Could you check a few things on this model? Use its own coordinates, in mm. Face numbers are marked on the shaded views. A direction names the side the tool comes from. Coordinates: 2 decimals unless noted, no trailing zeros.
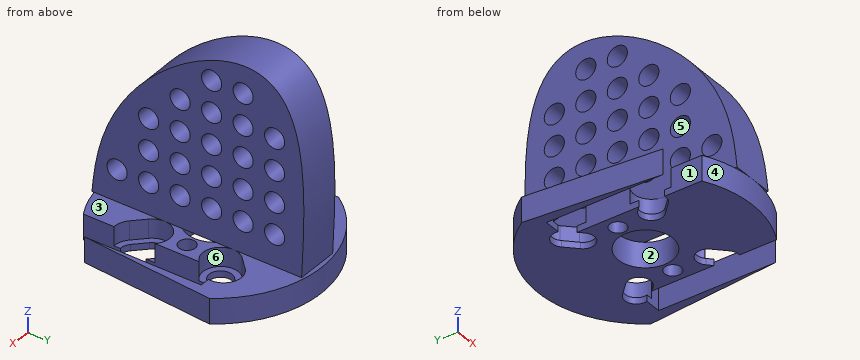
```python
from build123d import *

# Parameters (mm, degrees)
SKETCH_2_R          = 1.3
SKETCH_2_R_2        = 4.3
EXTRUDE_1_DEPTH     = 4
CUT_EXTRUDE_1_DEPTH = 3
EXTRUDE_START       = -3.4
EXTRUDE_2_DEPTH     = 6.8
CUT_EXTRUDE_START   = 3.4
SKETCH_12_R         = 1.6
CUT_EXTRUDE_2_DEPTH = 44.412015776


# Read off the part's stored shape, not the designer's step: 凸台-拉伸2
with BuildPart() as part:
    # 草图2 → 凸台-拉伸1 (new body)
    with BuildSketch(Plane.XY):
        with BuildLine():
            Line((-14.150895062, 9.420836955), (-12.3, -11.734990413))
            Line((-12.3, -11.734990413), (-12.3, 6.8))
            Line((-12.3, 6.8), (-9.717210306, 6.8))
            ThreePointArc((-9.717210306, 6.8), (-8.843521096, 8.787489117), (-6.693130483, 8.488714895))
            Line((-6.693130483, 8.488714895), (-4.92536353, 6.720947942))
            ThreePointArc((-4.92536353, 6.720947942), (-4.92536353, 4.17536353), (-7.470947942, 4.17536353))
            Line((-7.470947942, 4.17536353), (-8.2, 4.904415588))
            Line((-8.2, 4.904415588), (-8.2, -4.904415588))
            Line((-8.2, -4.904415588), (-7.470947942, -4.17536353))
            ThreePointArc((-7.470947942, -4.17536353), (-4.92536353, -4.17536353), (-4.92536353, -6.720947942))
            Line((-4.92536353, -6.720947942), (-6.693130483, -8.488714895))
            ThreePointArc((-6.693130483, -8.488714895), (-7.386916292, -8.92025587), (-8.2, -9.00063774))
            Line((-8.2, -9.00063774), (-8.2, -14.891608375))
            ThreePointArc((-8.2, -14.891608375), (0, -17), (8.2, -14.891608375))
            Line((8.2, -14.891608375), (8.2, -9.00063774))
            ThreePointArc((8.2, -9.00063774), (7.386916292, -8.92025587), (6.693130483, -8.488714895))
            Line((6.693130483, -8.488714895), (4.92536353, -6.720947942))
            ThreePointArc((4.92536353, -6.720947942), (4.92536353, -4.17536353), (7.470947942, -4.17536353))
            Line((7.470947942, -4.17536353), (8.2, -4.904415588))
            Line((8.2, -4.904415588), (8.2, 4.904415588))
            Line((8.2, 4.904415588), (7.470947942, 4.17536353))
            ThreePointArc((7.470947942, 4.17536353), (4.92536353, 4.17536353), (4.92536353, 6.720947942))
            Line((4.92536353, 6.720947942), (6.693130483, 8.488714895))
            ThreePointArc((6.693130483, 8.488714895), (8.843521096, 8.787489117), (9.717210306, 6.8))
            Line((9.717210306, 6.8), (12.3, 6.8))
            Line((12.3, 6.8), (12.3, -11.734990413))
            Line((12.3, -11.734990413), (14.150895062, 9.420836955))
            ThreePointArc((14.150895062, 9.420836955), (0, 17), (-14.150895062, 9.420836955))
        make_face()
        with Locations((-6, 0)):
            Circle(SKETCH_2_R, mode=Mode.SUBTRACT)
        Circle(SKETCH_2_R_2, mode=Mode.SUBTRACT)
        with Locations((6, 0)):
            Circle(SKETCH_2_R, mode=Mode.SUBTRACT)
    extrude(amount=EXTRUDE_1_DEPTH)

    # 草图10 → 切除-拉伸1 (cut)
    with BuildSketch(Plane.XY.offset(4)):
        with BuildLine():
            Line((-5.986023702, 9.195821676), (-4.218256749, 7.428054723))
            ThreePointArc((-4.218256749, 7.428054723), (-4.218256749, 3.468256749), (-8.178054723, 3.468256749))
            Line((-8.178054723, 3.468256749), (-9.945821676, 5.236023702))
            ThreePointArc((-9.945821676, 5.236023702), (-9.945821676, 9.195821676), (-5.986023702, 9.195821676))
        make_face()
        with BuildLine():
            Line((-5.986023702, -9.195821676), (-4.218256749, -7.428054723))
            ThreePointArc((-4.218256749, -7.428054723), (-4.218256749, -3.468256749), (-8.178054723, -3.468256749))
            Line((-8.178054723, -3.468256749), (-9.945821676, -5.236023702))
            ThreePointArc((-9.945821676, -5.236023702), (-9.945821676, -9.195821676), (-5.986023702, -9.195821676))
        make_face()
        with BuildLine():
            Line((5.986023702, 9.195821676), (4.218256749, 7.428054723))
            ThreePointArc((4.218256749, 7.428054723), (4.218256749, 3.468256749), (8.178054723, 3.468256749))
            Line((8.178054723, 3.468256749), (9.945821676, 5.236023702))
            ThreePointArc((9.945821676, 5.236023702), (9.945821676, 9.195821676), (5.986023702, 9.195821676))
        make_face()
        with BuildLine():
            Line((5.986023702, -9.195821676), (4.218256749, -7.428054723))
            ThreePointArc((4.218256749, -7.428054723), (4.218256749, -3.468256749), (8.178054723, -3.468256749))
            Line((8.178054723, -3.468256749), (9.945821676, -5.236023702))
            ThreePointArc((9.945821676, -5.236023702), (9.945821676, -9.195821676), (5.986023702, -9.195821676))
        make_face()
    extrude(amount=-CUT_EXTRUDE_1_DEPTH, mode=Mode.SUBTRACT)

    # 凸台-拉伸2 outline → 凸台-拉伸2 (add)
    with BuildSketch(Plane(origin=(0, 0, 0), x_dir=(0, 0, -1), z_dir=(1, 0, 0)).offset(EXTRUDE_START)):
        with BuildLine():
            Line((-4, -17), (-4, 16.2788168))
            add(Edge.make_bspline(
                [(-4, 16.2788168), (-25.43589952, 17.477300344), (-46.149481519, 17.5570925), (-34, 4.437094901), (-30.42433351, -15.568255951), (-11.367420307, -16.201944254), (-4, -17)],
                knots=[0, 0, 0, 0, 0, 0, 0, 1, 1, 1, 1, 1, 1, 1], degree=6))
        make_face()
    extrude(amount=EXTRUDE_2_DEPTH)

    # 草图12 → 切除-拉伸2 (cut, through all)
    with BuildSketch(Plane(origin=(0, 0, 0), x_dir=(0, 0, -1), z_dir=(1, 0, 0)).offset(CUT_EXTRUDE_START)):
        with Locations((-9, 12)):
            Circle(SKETCH_12_R)
        with Locations((-9, -13)):
            Circle(SKETCH_12_R)
        with Locations((-9, 7)):
            Circle(SKETCH_12_R)
        with Locations((-9, -8)):
            Circle(SKETCH_12_R)
        with Locations((-9, 2)):
            Circle(SKETCH_12_R)
        with Locations((-9, -3)):
            Circle(SKETCH_12_R)
        with Locations((-29, 7)):
            Circle(SKETCH_12_R)
        with Locations((-29, 2)):
            Circle(SKETCH_12_R)
        with Locations((-24, 12)):
            Circle(SKETCH_12_R)
        with Locations((-19, 12)):
            Circle(SKETCH_12_R)
        with Locations((-14, 12)):
            Circle(SKETCH_12_R)
        with Locations((-24, 7)):
            Circle(SKETCH_12_R)
        with Locations((-19, 7)):
            Circle(SKETCH_12_R)
        with Locations((-14, 7)):
            Circle(SKETCH_12_R)
        with Locations((-24, 2)):
            Circle(SKETCH_12_R)
        with Locations((-19, 2)):
            Circle(SKETCH_12_R)
        with Locations((-14, 2)):
            Circle(SKETCH_12_R)
        with Locations((-24, -3)):
            Circle(SKETCH_12_R)
        with Locations((-19, -3)):
            Circle(SKETCH_12_R)
        with Locations((-14, -3)):
            Circle(SKETCH_12_R)
        with Locations((-19, -8)):
            Circle(SKETCH_12_R)
        with Locations((-14, -8)):
            Circle(SKETCH_12_R)
    extrude(amount=-CUT_EXTRUDE_2_DEPTH, mode=Mode.SUBTRACT)


solid = part.part
```
1. Please list where these lines run through material, in increasing order: line 1 along Y through (x, z) = (-1.75, 19); line 2 along Z through (x, y) = (0.25, -2); line 3 along Y through (x, z) = (0.75, 14).
Verdict:
line 1: y = -12.71 to -9.6, -6.4 to -4.6, -1.4 to 0.4, 3.6 to 5.4, 8.6 to 10.4, 13.6 to 16.5
line 2: z = 4 to 7.75, 10.25 to 12.75, 15.25 to 17.75, 20.25 to 22.75, 25.25 to 30.1
line 3: y = -15.03 to -9.6, -6.4 to -4.6, -1.4 to 0.4, 3.6 to 5.4, 8.6 to 10.4, 13.6 to 16.63
2. If we mould it in two halves opening along X, with no side actions, what happens to the marked faces 4, 5 and 6? For each: pulls with the +X half, pulls with the -X half, needs draft (parallel to the pull), parting line crosses it, or undercut.
Verdict:
face 4: parting line crosses it
face 5: needs draft
face 6: undercut
3. For pin 1 (4 mm diameter, centred on x = 0.5, z = 17.5, fed in from +Y); pin 2 (5 mm diameter, centred on y = 7, z = 9, fed in from +X); pin 3 (4 mm diameter, centred on y = -8.5, z = 28, fed in from +X); pin 4 (2 mm diameter, centred on y = -11.5, z = 2, fed in from +X), each with a flat end and sliding along its axis, tell me the tip position at first contact or that it passes through.
Verdict:
pin 1: stops at y = 16.63
pin 2: stops at x = 3.4
pin 3: passes through
pin 4: stops at x = 12.41
4. On a 3-axis mill with a long thin cutter (end or side, diameter ignored), from which of +Z, -Z, +X, -X, +Y, -Y can I reach the whole of each face in a straight line? I mean the marked faces 1, 2 and 3. Say none if no direction works.
Verdict:
face 1: +Z, -Z, -Y
face 2: -Z
face 3: +Z, +X, +Y, -Y
5. I want a section at A-A on z = 14. Give the number of separate pieces and of enclosed holes in the cut face, plus the area to 3 significant figures.
Verdict:
separate pieces: 6
enclosed holes: 0
area: 106 mm2
